For this review, take the finished solid that the model builds, in its own axes (mm). Face numbers are marked on the shaded views. A direction names the side the tool comes from. Give positions to 0.01 mm unless a question says otherwise; leave off trailing zeros. Order: outer loops, then holes, each group sorted by start corner. A loop starts at its lowest first (then second) coordinate and runs counter-clockwise, first axis right, second up. Notation, with made-up numbers: (-37, 54.5) - (8, 54.5) arc R23 cw to (8, 70.5) - close; hole circle Ø10 at (56.25, 75.25). An arc over 180 degrees is marked (long way). Answer as a JSON object with one key per item and string values. Group by question number.
Autodesk Inventor part; units mm, degrees
ref_plane "Plano de trabajo1" through (0, 0, 50) normal (0, 0, -1) x (-1, 0, 0)
ref_plane "YZ Plane" through (0, 0, 0) normal (1, 0, 0) x (0, 1, 0)
ref_plane "XZ Plane" through (0, 0, 0) normal (0, 1, 0) x (-1, 0, 0)
sketch "Boceto2" plane through (0, 0, 0) normal (0, 0, 1) x (1, 0, 0)
  circle A0 centre (-16.7491, 0.2224) radius 9
  circle A1 centre (138.5611, 0.2224) radius 9
  line L0 (-9.2658, 5.2224) -> (131.0778, 5.2224)
  line L1 (131.0778, -4.7776) -> (-9.2658, -4.7776)
  circle A2 centre (138.5611, 0.2224) radius 5
  circle A3 centre (-16.7491, 0.2224) radius 5
  point P0 (0, 0)
  dimension "d2" = 18
  dimension "d3" = 10
  dimension "d4" = 10
extrude "Extrusión1" add sketch "Boceto2" along normal blind 100 contours A0 L0 A1 L1
ref_plane "Plano de trabajo1" through (0, 0, 50) normal (0, 0, -1) x (-1, 0, 0)
sketch "Boceto3" plane through (0, 0, 50) normal (0, 0, -1) x (-1, 0, 0)
  circle A0 centre (-138.5611, 0.2224) radius 9
  circle A1 centre (16.7491, 0.2224) radius 9
  circle A2 centre (-138.5611, 0.2224) radius 5
  circle A3 centre (16.7491, 0.2224) radius 5
  point P0 (0, 0)
extrude "Extrusión2" add sketch "Boceto3" along normal mid plane 105
sketch "Boceto4" plane through (0, 0, 0) normal (0, 1, 0) x (-1, 0, 0)
  line L0 (25.7491, 102.5) -> (25.7491, -2.5)
  line L1 (9.2658, 0) -> (-131.0778, 0)
  line L2 (9.2658, 100) -> (-131.0778, 100)
  line L3 (-147.5611, 102.5) -> (-147.5611, -2.5)
  line L4 (25.7491, 9) -> (-14.9531, 9)
  line L5 (-14.9531, 9) -> (-57.3933, 0)
  line L6 (9.2658, 0) -> (-131.0778, 0)
  line L7 (-57.3933, 100) -> (-14.9531, 91)
  line L8 (-14.9531, 91) -> (25.7491, 91)
  line L9 (25.7491, 75) -> (-8.8807, 75)
  line L10 (-8.8807, 75) -> (-8.8807, 25)
  line L11 (-8.8807, 25) -> (25.7491, 25)
  line L12 (-24.9356, 70.614) -> (-24.9356, 29.386)
  line L13 (-83.4051, 51.7146) -> (-115.5189, 73.8108)
  line L14 (-118.6526, 72.1632) -> (-118.6526, 61.0832)
  line L15 (-118.6526, 39.8101) -> (-118.6526, 28.73)
  line L16 (-115.5457, 27.0642) -> (-83.4319, 48.4011)
  line L17 (-28.4456, 71.9255) -> (-48.8564, 48.4239)
  line L18 (-28.247, 27.8759) -> (-48.6578, 45.6025)
  line L19 (-57.9307, 80) -> (-88.0143, 80) construction
  line L20 (-57.9307, 89.5575) -> (-88.0143, 89.5575)
  line L21 (-88.0143, 70.4425) -> (-57.9307, 70.4425)
  arc A0 (-57.9307, 70.4425) -> (-57.9307, 89.5575) centre (-57.9307, 80) ccw
  arc A1 (-88.0143, 89.5575) -> (-88.0143, 70.4425) centre (-88.0143, 80) ccw
  line L22 (-57.9307, 18.0061) -> (-88.508, 18.0061) construction
  line L23 (-57.9307, 27.6984) -> (-88.508, 27.6984)
  line L24 (-88.508, 8.3137) -> (-57.9307, 8.3137)
  arc A2 (-57.9307, 8.3137) -> (-57.9307, 27.6984) centre (-57.9307, 18.0061) ccw
  arc A3 (-88.508, 27.6984) -> (-88.508, 8.3137) centre (-88.508, 18.0061) ccw
  line L25 (-118.6526, 61.0832) -> (-103.6526, 55.6402)
  arc A4 (-105.6651, 44.0001) -> (-103.6526, 55.6402) centre (-105.6992, 50) ccw
  line L26 (-105.6651, 44.0001) -> (-117.037, 41.7728)
  arc A5 (-115.5189, 73.8108) -> (-118.6526, 72.1632) centre (-116.6526, 72.1632) ccw
  arc A6 (-83.4319, 48.4011) -> (-83.4051, 51.7146) centre (-84.5388, 50.0669) ccw
  arc A7 (-118.6526, 28.73) -> (-115.5457, 27.0642) centre (-116.6526, 28.73) ccw
  arc A8 (-117.037, 41.7728) -> (-118.6526, 39.8101) centre (-116.6526, 39.8101) ccw
  arc A9 (-28.247, 27.8759) -> (-24.9356, 29.386) centre (-26.9356, 29.386) ccw
  arc A10 (-24.9356, 70.614) -> (-28.4456, 71.9255) centre (-26.9356, 70.614) ccw
  arc A11 (-48.8564, 48.4239) -> (-48.6578, 45.6025) centre (-47.3464, 47.1125) ccw
  line L27 (25.7491, 100) -> (25.7491, 91)
  line L28 (7.7491, 102.5) -> (7.7491, -2.5)
  line L29 (-57.3933, 100) -> (7.7491, 100)
  line L30 (7.7491, 102.5) -> (25.7491, 102.5)
  line L31 (25.7491, 102.5) -> (7.7491, 102.5)
  point P0 (0, 0)
  point P1 (-24.9356, 75.967)
  point P2 (-24.9356, 25)
  point P3 (-80.9683, 50.038)
  point P4 (-118.6526, 75.967)
  point P5 (-118.6526, 41.4563)
  point P6 (-118.6526, 25)
  point P7 (-8.8807, 50)
  point P8 (25.7491, 50)
  point P9 (-24.9356, 50)
  point P10 (-50.1679, 46.9139)
  point P11 (-72.9725, 80)
  point P12 (-73.2193, 18.0061)
  point P13 (-147.5611, 50)
  dimension "d11" = 50
  dimension "d12" = 16
  dimension "d14" = 16
  dimension "d26" = 2
  dimension "d27" = 2
  dimension "d28" = 6
  dimension "d29" = 15
extrude "Extrusión4" cut sketch "Boceto4" along normal through all both and the other way through all contours L0 L8 L28 L30 | L28 L8 L7 L2 | L0 L11 L28 L9 | L28 L11 L10 L9 | L12 A9 L18 A11 L17 A10 | A6 L16 A7 L15 A8 L26 A4 L25 L14 A5 L13 | A0 L21 A1 L20 | A2 L24 A3 L23
sketch "Boceto5" plane through (57.9307, 5.2224, 8.3137) normal (0, 0, 1) x (1, 0, 0)
  line L0 (0, 0) -> (30.5774, 0)
  line L1 (0, -10) -> (0, 0)
  line L2 (30.5774, -10) -> (0, -10)
  line L3 (30.5774, -10) -> (30.5774, 0)
  circle A0 centre (15.2887, -5) radius 3
  line L4 (0, 0) -> (30.5774, 0)
  line L5 (0, -10) -> (0, 0)
  point P0 (-57.9307, -5.2224)
  point P1 (15.2887, 0)
  point P2 (0, -5)
  dimension "d32" = 6
extrude "Extrusión5" cut sketch "Boceto5" against normal through all contours A0
properties part number "Left_upper_part" material "Acero, suave"
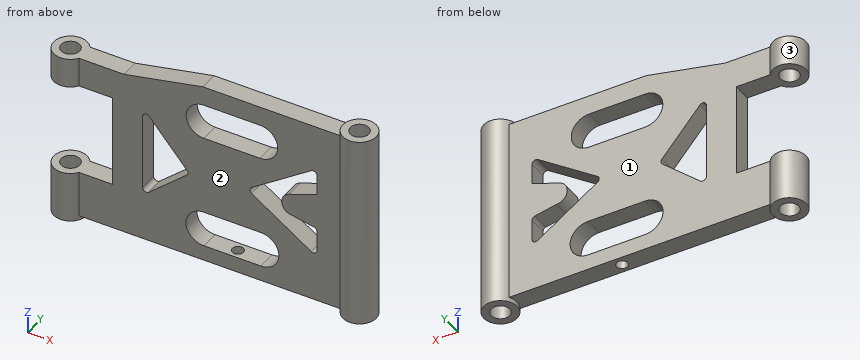
1) Consider section A-A (x = -1). Give the boundary of the cut face in (y, z).
2) For the marked faces 1, 2 and 3, list the 3-axis set-ups (+Z, -Z, +X, -X, +Y, -Y) from which the entire face can be reached by the end or side of a thin tool; tool diameter is ignored.
3) For pin 1 (5 mm diameter, centred on x = 58, y = 1.5, fed in from +Z); pin 2 (5 mm diameter, centred on x = 57.5, y = 0, fed in from -Z); pin 3 (8 mm diameter, centred on x = 3.5, z = 76.5, fed in from +Y), all flat-tipped, find the tip position at first contact; note any pin that passes through.
4) Consider section D-D (x = 34). Give the boundary of the cut face in (y, z), plus the area to 3 significant figures.
5) For line 1 (Z direction, x = 67, y = 3.75); line 2 (X direction, y = 3.25, z = 79.5); line 3 (X direction, y = -1, z = 5.5), list the stretches that pass through material, from the lowest coordinate up.
6) Consider section B-B (z = 79.5). Give the boundary of the cut face in (x, y).
7) Consider section C-C (y = 7.25). Give the boundary of the cut face in (x, z).
Result set:
{
 "1": {"outline": "(-4.78, 0) - (5.22, 0) - (5.22, 25) - (-4.78, 25) - close; (-4.78, 75) - (5.22, 75) - (5.22, 91) - (-4.78, 91) - close"},
 "2": {"face 1": "+Z, -Z, +Y", "face 2": "+Z, -Z, -Y", "face 3": "+Z, -Z"},
 "3": {"pin 1": "stops at z = 100", "pin 2": "stops at z = 0", "pin 3": "stops at y = 5.22"},
 "4": {"outline": "(-4.78, 0) - (5.22, 0) - (5.22, 32.87) - (-4.78, 32.87) - close; (-4.78, 65.53) - (5.22, 65.53) - (5.22, 95.04) - (-4.78, 95.04) - close", "area": "624 mm2"},
 "5": {"line 1": "z = 0 to 8.31, 27.7 to 70.44, 89.56 to 100", "line 2": "x = -25.22 to -20.73, -12.77 to 48.39, 97.56 to 134.58, 142.54 to 147.04", "line 3": "x = -25.67 to -21.6, -11.9 to 70.48, 75.96 to 133.71, 143.41 to 147.48"},
 "6": {"outline": "(-9.27, -4.78) - (48.39, -4.78) - (48.39, 5.22) - (-9.27, 5.22) arc R9 ccw (long way) to start; (97.56, -4.78) - (131.08, -4.78) arc R9 ccw (long way) to (131.08, 5.22) - (97.56, 5.22) - close; hole circle Ø10 at (-16.75, 0.22); hole circle Ø10 at (138.56, 0.22)"},
 "7": {"outline": "(-22.37, -2.5) - (-11.13, -2.5) - (-11.13, 25) - (-22.37, 25) - close; (-22.37, 75) - (-11.13, 75) - (-11.13, 91) - (-22.37, 91) - close; (132.94, -2.5) - (144.18, -2.5) - (144.18, 102.5) - (132.94, 102.5) - close"}
}
